Geometry: final body of the model. Coordinates: model frame, mm. A direction names the side the tool comes from. Round coordinates to 2 decimals unless told otherwise and drop trailing zeros. Order: outer loops, then holes, each group sorted by start corner. A loop starts at its lowest first (then second) coordinate and runs counter-clockwise, first axis right, second up. Notation, with made-up numbers: M 54,8 L 65,8 A19 cw 65,21 Z; hole C -15.5,13.5 d11. An arc over 180 degrees is marked long. Put each result on its own line as item: value. Start each with the question number.
1) Draft query along Z for faces 1 (the cylindrical face through (23.835, 18.054, 21.986)), 2 (the cylindrical face through (1.61, 12.979, 209.544)), 3 (the flat face through (24, 13, 0)), 4 (the flat face through (13, 25.4, 113)). Return one class per face: pulls with the +Z half, pulls with the -Z half, needs draft (parallel to the pull), parting line crosses it, or undercut.
2) Section B-B, the plane y = 12.7. Return loops of the section in (x, z) (3 decimals), then the cut area to 3 significant figures.
3) Section C-C, the plane x = 20. Return loops of the section in (y, z) (3 decimals).
4) Access query for faces 5 (the flat face through (3.175, 13, 113)), 6 (the cylindrical face through (1.61, 18.054, 21.986)). Directions: +Z, -Z, +X, -X, +Y, -Y. A direction counts if a zero-diameter tool reaches every point of the face in a straight line with its end or side. Return the directions, or none.
5) Section A-A, the plane z = 125.5. Return loops of the section in (x, y) (3 decimals), then the cut area to 3 significant figures.
6) Material intervals for probe 1 along X at (y, z) = (4, 126.5) (3 decimals); probe 2 along Y at (x, z) = (23.05, 203.2), sorted ascending. Write a range as [from, to].
7) First-contact query: P1, Ø10, axis at x = 3.5, z = 96, coming from the -Y side; P2, Ø7.5, axis at y = 12.7, z = 25.4, coming from the -X side (3 decimals). Flat tips, straight axial feed; report the tip coordinate or a pass-through.
8) Section D-D, the plane z = 203.2. Return loops of the section in (x, y) (3 decimals).
Autodesk Inventor part; units mm, degrees
ref_plane "YZ Plane" through (0, 0, 0) normal (1, 0, 0) x (0, 1, 0)
ref_plane "XZ Plane" through (0, 0, 0) normal (0, 1, 0) x (-1, 0, 0)
ref_plane "XY Plane" through (0, 0, 0) normal (0, 0, 1) x (1, 0, 0)
sketch "Sketch1" plane through (0, 0, 0) normal (0, 0, 1) x (1, 0, 0)
  line L0 (0, 0) -> (25.4, 0)
  line L1 (25.4, 0) -> (25.4, 25.4)
  line L2 (25.4, 25.4) -> (0, 25.4)
  line L3 (0, 25.4) -> (0, 0)
  dimension "d0" = 25.4
  dimension "d1" = 25.4
extrude "Extrusion1" add sketch "Sketch1" along normal blind 228.6
shell "Shell1" thickness 3.175 removed faces 2 at (8.4667, 16.9333, 0) at (8.4667, 16.9333, 228.6)
sketch "Sketch2" plane through (25.4, 0, 0) normal (1, 0, 0) x (0, 0, -1)
  circle A0 centre (-25.4, 12.7) radius 6.35
  line L0 (0, 25.4) -> (-228.6, 25.4)
  line L1 (0, 0) -> (0, 25.4)
  circle A1 centre (-203.2, 12.7) radius 6.35
  line L2 (-228.6, 0) -> (-228.6, 25.4)
  dimension "d5" = 12.7
  dimension "d6" = 12.7
  dimension "d7" = 25.4
  dimension "d10" = 12.7
  dimension "d11" = 12.7
  dimension "d12" = 25.4
extrude "Extrusion2" cut sketch "Sketch2" against normal blind 228.6
properties part number "Kermit Arm_Connecter"
Result sheet:
1. face 1: undercut
1. face 2: undercut
1. face 3: pulls with the -Z half
1. face 4: needs draft
2. outline: M 0,0 L 3.175,0 L 3.175,19.05 L 0,19.05 Z; M 0,31.75 L 3.175,31.75 L 3.175,196.85 L 0,196.85 Z; M 0,209.55 L 3.175,209.55 L 3.175,228.6 L 0,228.6 Z; M 22.225,0 L 25.4,0 L 25.4,19.05 L 22.225,19.05 Z; M 22.225,31.75 L 25.4,31.75 L 25.4,196.85 L 22.225,196.85 Z; M 22.225,209.55 L 25.4,209.55 L 25.4,228.6 L 22.225,228.6 Z
2. area: 1,290 mm2
3. outline: M 0,0 L 3.175,0 L 3.175,228.6 L 0,228.6 Z; M 22.225,0 L 25.4,0 L 25.4,228.6 L 22.225,228.6 Z
4. face 5: +Z, -Z
4. face 6: +X, -X
5. outline: M 0,0 L 25.4,0 L 25.4,25.4 L 0,25.4 Z; hole M 3.175,3.175 L 22.225,3.175 L 22.225,22.225 L 3.175,22.225 Z
5. area: 282 mm2
6. probe 1: x = [0, 3.175], [22.225, 25.4]
6. probe 2: y = [0, 6.35], [19.05, 25.4]
7. P1: stops at y = 0
7. P2: passes through
8. outline: M 0,0 L 25.4,0 L 25.4,6.35 L 22.225,6.35 L 22.225,3.175 L 3.175,3.175 L 3.175,6.35 L 0,6.35 Z; M 0,19.05 L 3.175,19.05 L 3.175,22.225 L 22.225,22.225 L 22.225,19.05 L 25.4,19.05 L 25.4,25.4 L 0,25.4 Z
